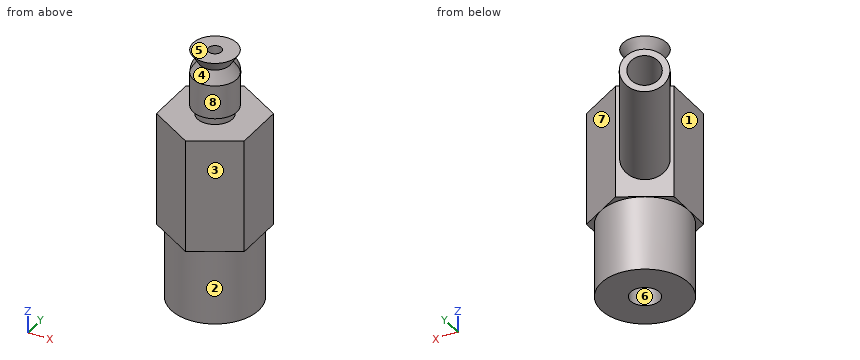
```python
from build123d import *

# Parameters (mm, degrees)
SKETCH_1_R             = 5
EXTRUDE_1_DEPTH        = 8.5
EXTRUDE_2_DEPTH        = 13
SKETCH_3_R             = 2
EXTRUDE_3_DEPTH        = 1
SKETCH_5_R             = 0.75
CUT_EXTRUDE_1_DEPTH    = 15
SKETCH_6_R             = 2.5
EXTRUDE_4_DEPTH        = 16
SKETCH_7_R             = 1.75
CUT_EXTRUDE_2_DEPTH    = 22
HOLE_WIZARD_M4_1_D     = 3.3
HOLE_WIZARD_M4_1_DEPTH = 10.1
HOLE_WIZARD_M4_1_TIP   = 0.991420021


with BuildPart() as part:
    # 草图1 → 凸台-拉伸1 (new body)
    with BuildSketch(Plane.XY):
        Circle(SKETCH_1_R)
    extrude(amount=EXTRUDE_1_DEPTH)

    # 草图2 → 凸台-拉伸2 (add)
    with BuildSketch(Plane.XY.offset(8.5)):
        Polygon((5, 2.886751346), (0, 5.773502692), (-5, 2.886751346), (-5, -2.886751346), (0, -5.773502692), (5, -2.886751346), align=None)
    extrude(amount=EXTRUDE_2_DEPTH)

    # 草图3 → 凸台-拉伸3 (add)
    with BuildSketch(Plane.XY.offset(21.5)):
        Circle(SKETCH_3_R)
    extrude(amount=EXTRUDE_3_DEPTH)

    # 草图4 → 旋转1 (revolve)
    with BuildSketch(Plane(origin=(0, 0, 0), x_dir=(1, 0, 0), z_dir=(0, 1, 0)), mode=Mode.PRIVATE) as revolve_1_sk:
        Polygon((0, -22.5), (2.5, -22.5), (2.5, -26.347532538), (1.664204883, -27.683358747), (2.5, -29), (0, -29), align=None)
    revolve(revolve_1_sk.sketch.rotate(Axis((0, 0, 22.5), (0, 0, 1)), 180), axis=Axis((0, 0, 22.5), (0, 0, 1)))

    # 草图5 → 切除-拉伸1 (cut)
    with BuildSketch(Plane.XY.offset(29)):
        Circle(SKETCH_5_R)
    extrude(amount=-CUT_EXTRUDE_1_DEPTH, mode=Mode.SUBTRACT)

    # 草图6 → 凸台-拉伸4 (add)
    with BuildSketch(Plane(origin=(-2.5, 4.330127019, 0), x_dir=(0.8660254037844388, 0.49999999999999983, 0), z_dir=(-0.4999999999999998, 0.8660254037844387, 0))):
        with Locations((0, -13)):
            Circle(SKETCH_6_R)
    extrude(amount=EXTRUDE_4_DEPTH)

    # 草图7 → 切除-拉伸2 (cut)
    with BuildSketch(Plane(origin=(-10.5, 18.186533479, 0), x_dir=(0.8660254037844387, 0.49999999999999994, 0), z_dir=(-0.4999999999999999, 0.8660254037844386, 0))):
        with Locations(Location((0, -13, 0), (0, 0, 180))):
            Circle(SKETCH_7_R)
    extrude(amount=-CUT_EXTRUDE_2_DEPTH, mode=Mode.SUBTRACT)

    # M4 螺纹孔1
    with Locations(Plane(origin=(0, 0, 0), x_dir=(-1, 0, 0), z_dir=(0, 0, -1))):
        with Locations((0, 0)):
            Hole(HOLE_WIZARD_M4_1_D / 2, depth=HOLE_WIZARD_M4_1_DEPTH)
            with Locations((0, 0, -(HOLE_WIZARD_M4_1_DEPTH + HOLE_WIZARD_M4_1_TIP / 2))):  # 118° drill point
                Cone(0, HOLE_WIZARD_M4_1_D / 2, HOLE_WIZARD_M4_1_TIP, mode=Mode.SUBTRACT)


solid = part.part
```
Input: part model. Units: mm. Frame: model coordinates. Face numbers are marked on the shaded views. A direction names the side the tool comes from. Round coordinates to 2 decimals unless told otherwise and drop trailing zeros. Loops run counter-clockwise (first coordinate to the right, second up) from the corner with the lowest first, then second, coordinate; pieces in that order, holes last.
1) Material intervals for line 1 (Y direction, x = 0, z = 8); line 2 (X direction, y = 0, z = 17.5); line 3 (Z direction, x = 2.75, y = 3), sorted ascending.
Ans:
line 1: y = -5 to -1.65, 1.65 to 5
line 2: x = -5 to -0.75, 0.75 to 5
line 3: z = 0 to 21.5
2) Pull-direction query (X, two-part tool) for the marked faces 6, 7 and 8; classes: released by +X, released by -X, zero draft, split by the parting line, or undercut.
Ans:
face 6: undercut
face 7: released by +X
face 8: split by the parting line
3) Section query D-D on z = 5.5. Return the cut outline in (x, y).
Ans:
outline: circle Ø10 at (0, 0); hole circle Ø3.3 at (0, 0)
4) Pin query (flat end, axial travel): pin 1 (6.5 mm diameter, centred on y = 0, z = 16.5, fed in from -X); pin 2 (2 mm diameter, centred on x = 0, y = 0, fed in from -Z); pin 3 (1.5 mm diameter, centred on x = 0, y = 0, fed in from -Z); pin 4 (1.5 mm diameter, centred on x = -4, z = 24, fed in from +Y). Return the tip coordinate at first contact, or that it passes through.
Ans:
pin 1: stops at x = -5
pin 2: stops at z = 10.49
pin 3: stops at z = 10.64
pin 4: passes through
5) Section query C-C on x = 3. Return the cut outline in (y, z).
Ans:
outline: (-4.04, 8.5) - (-4, 8.5) - (-4, 0) - (4, 0) - (4, 8.5) - (4.04, 8.5) - (4.04, 21.5) - (-4.04, 21.5) - close
6) Section query A-A on z = 9.25. Return the cut outline in (x, y).
Ans:
outline: (-5, -2.89) - (0, -5.77) - (5, -2.89) - (5, 2.89) - (0, 5.77) - (-5, 2.89) - close; hole circle Ø3.3 at (0, 0)
7) Section query B-B on z = 18.25. Return the cut outline in (x, y), plus the area to 3 significant figures.
Ans:
outline: (-5, -2.89) - (0, -5.77) - (5, -2.89) - (5, 2.89) - (0, 5.77) - (-5, 2.89) - close; hole circle Ø1.5 at (0, 0)
area: 84.8 mm2
8) Set-up query: the marked faces 1, 2, 3, 4 and 5. Return all of +Z, -Z, +X, -X, +Y, -Y with unobstructed straight access to the full face (end or side cutting, diameter ignored); none if empty.
Ans:
face 1: +Z, -Z, -X, -Y
face 2: -Z
face 3: +Z, -Z, +X, -Y
face 4: none
face 5: +Z, +X, -X, +Y, -Y
